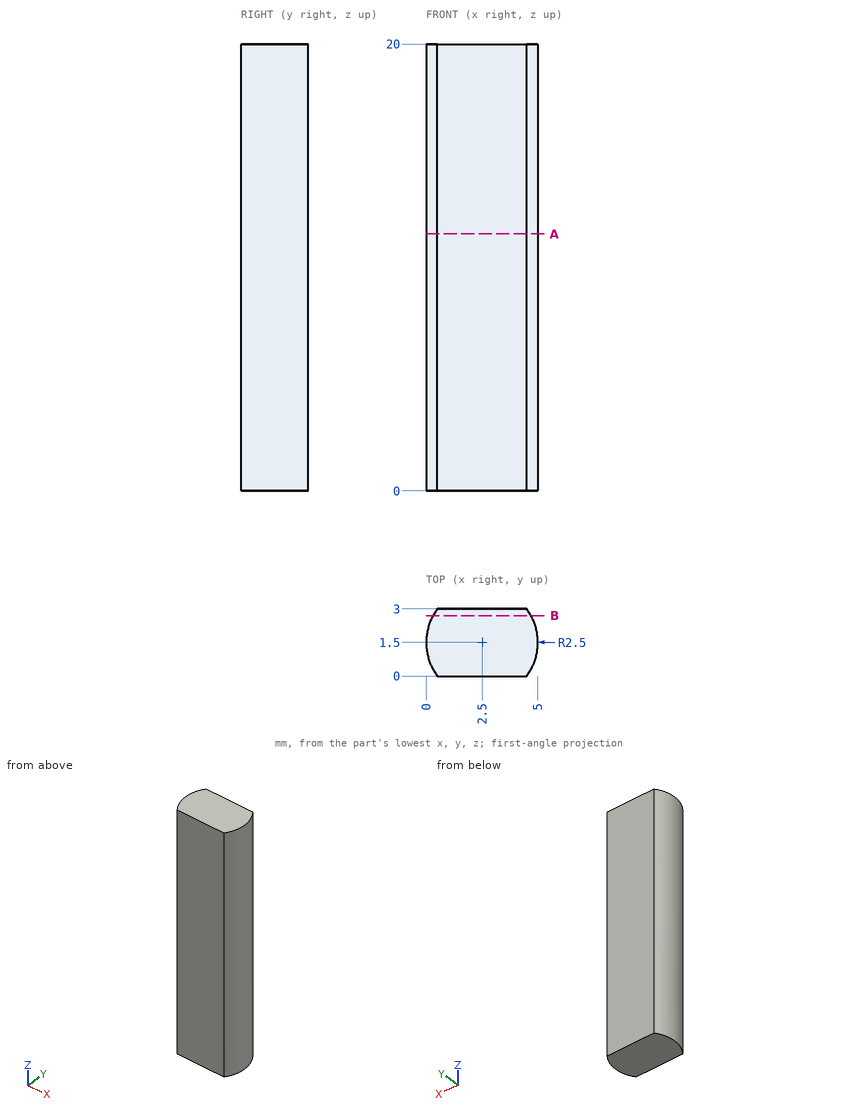
Here's the drawing with two shaded views (mm, measured from the low corner). I have some questions. Give positions to 0.01 mm unless a question says otherwise; leave off trailing zeros. Order: outer loops, then holes, each group sorted by start corner. A loop starts at its lowest first (then second) coordinate and runs counter-clockwise, first axis right, second up. Notation, with made-up numbers: (-19.5, 87.5) -> (16.5, 87.5) arc R15 ccw to (16.5, 98.5) -> close; hole circle Ø4 at (31, -20.75). An arc over 180 degrees is marked (long way). Use a Markdown table: item, result. Add a question column.
Item 1: I need wall thicknesses on line 1 (X direction, y = 1.4, z = 3); line 2 (Y direction, x = 0.45, z = 8.75); line 3 (X direction, y = 2.7, z = 11). Which ranges of each line are inside material? Lowest first, please.
Item 2: Imagine slicing it at A-A on z = 11.5. Please give me the cut outline in (x, y), plus the area to 3 significant figures.
Item 3: Imagine slicing it at B-B on y = 2.7. Please give me the cut outline in (x, z), plus the area to 3 significant figures.
Data:
| question | item | result |
|---|---|---|
| 1 | line 1 | x = 0 to 5 |
| 1 | line 2 | y = 0.07 to 2.93 |
| 1 | line 3 | x = 0.31 to 4.69 |
| 2 | outline | (0.5, 0) -> (4.5, 0) arc R2.5 ccw to (4.5, 3) -> (0.5, 3) arc R2.5 ccw to start |
| 2 | area | 14.0 mm² |
| 3 | outline | (0.31, 0) -> (4.69, 0) -> (4.69, 20) -> (0.31, 20) -> close |
| 3 | area | 87.7 mm² |
